For this review, take the finished solid that the model builds, in its own axes (mm). A direction names the side the tool comes from. Coordinates: 2 decimals unless noted, no trailing zeros. Write each loop counter-clockwise with the first axis right and the second up, starting at its lowest first coordinate (ties: lowest second). Pieces come first, ordered by that corner, then holes. Notation, with made-up numbers: (-15, 56.5) -> (22, 56.5) arc R24 ccw to (22, 88.5) -> close; hole circle Ø2 at (77.25, -35). An arc over 180 degrees is marked (long way). One line per item, written item: value. Start each with the question number.
1) For pin 1 Ø4 at (y, z) = (-3.5, 24.5) entering from +X; pin 2 Ø1 at (y, z) = (-5, 14) entering from -X; pin 3 Ø4 at (y, z) = (-7.5, 20.5) entering from +X, all flat-tipped, find the tip position at first contact; note any pin that passes through.
2) For probe 1 along Z at (x, y) = (-30.5, -0.25) (3 decimals); probe 2 along X at (y, z) = (-5.5, 18); probe 3 along X at (y, z) = (-8, 31.5), list the stretches that pass through material, from the lowest coordinate up. Write a range as from..to.
3) Add section A-A (x = -40). State the section outline as (y, z) points (3 decimals).
4) Machinability: for faces 1 (the flat face through (-26, -5, 6)), 2 (the flat face through (-24, -5, 34.925)), which of the approach directions +Z, -Z, +X, -X, +Y, -Y give a long, thin tool a straight path to every point of the face, cutting with its end or side? Answer none if there is none.
5) Add section C-C (z = 9). State the section outline as (x, y) points, and give its area (3 significant figures).
6) Add section B-B (y = -1.75). State the section outline as (x, z) points (1 decimal).
7) Add section D-D (z = 28). State the section outline as (x, y) points.
8) Mouldability with a two-part tool opening along Z and no side actions: class faces 3 (the flat face through (-22, -10, 5)), 4 (the flat face through (-26, -5, 30.53)), 5 (the flat face through (-24, -5, 0)) as released by +Z, released by -Z, zero draft, split by the parting line, or undercut.
from build123d import *

# Parameters (mm, degrees)
F1_DEPTH = 10


with BuildPart() as f1:
    # F0 (on Front) → F1 (new body)
    with BuildSketch(Plane.XZ):
        with BuildLine():
            Line((1.427054, 34.925), (-49.372946, 34.925))
            Line((-49.372946, 34.925), (-49.372946, 30.529865))
            Line((-49.372946, 30.529865), (-2.427831, 30.529865))
            ThreePointArc((-2.427831, 30.529865), (-0.638579, 32.848636), (1.427054, 34.925))
        make_face()
        with BuildLine():
            Line((-49.372946, 0), (1.427054, 0))
            ThreePointArc((1.427054, 0), (-1.246391, 2.798302), (-3.420543, 6))
            Line((-3.420543, 6), (-49.372946, 6))
            Line((-49.372946, 6), (-49.372946, 0))
        make_face()
        with BuildLine():
            ThreePointArc((1.427054, 0), (-2.517107, 17.4625), (1.427054, 34.925))
            ThreePointArc((1.427054, 34.925), (-0.638579, 32.848636), (-2.427831, 30.529865))
            ThreePointArc((-2.427831, 30.529865), (-6.410939, 18.40604), (-3.420543, 6))
            ThreePointArc((-3.420543, 6), (-1.246391, 2.798302), (1.427054, 0))
        make_face()
    extrude(amount=F1_DEPTH)


solid = f1.part
Numbers:
1. pin 1: x = -1.5
1. pin 2: x = -6.24
1. pin 3: x = -2.2
2. probe 1: 0..6, 30.53..34.925
2. probe 2: -6.42..-2.51
2. probe 3: -49.37..-0.02
3. outline: (-10, 0) -> (0, 0) -> (0, 6) -> (-10, 6) -> close; (-10, 30.53) -> (0, 30.53) -> (0, 34.925) -> (-10, 34.925) -> close
4. face 1: -X, +Y, -Y
4. face 2: +Z, +X, -X, +Y, -Y
5. outline: (-4.84, -10) -> (-1.63, -10) -> (-1.63, 0) -> (-4.84, 0) -> close
5. area: 32.2 mm²
6. outline: (-49.4, 0) -> (1.4, 0) arc R40.6 cw to (1.4, 34.9) -> (-49.4, 34.9) -> (-49.4, 30.5) -> (-2.4, 30.5) arc R23.3 ccw to (-3.4, 6) -> (-49.4, 6) -> close
7. outline: (-3.92, -10) -> (-1.13, -10) -> (-1.13, 0) -> (-3.92, 0) -> close
8. face 3: zero draft
8. face 4: undercut
8. face 5: released by -Z
